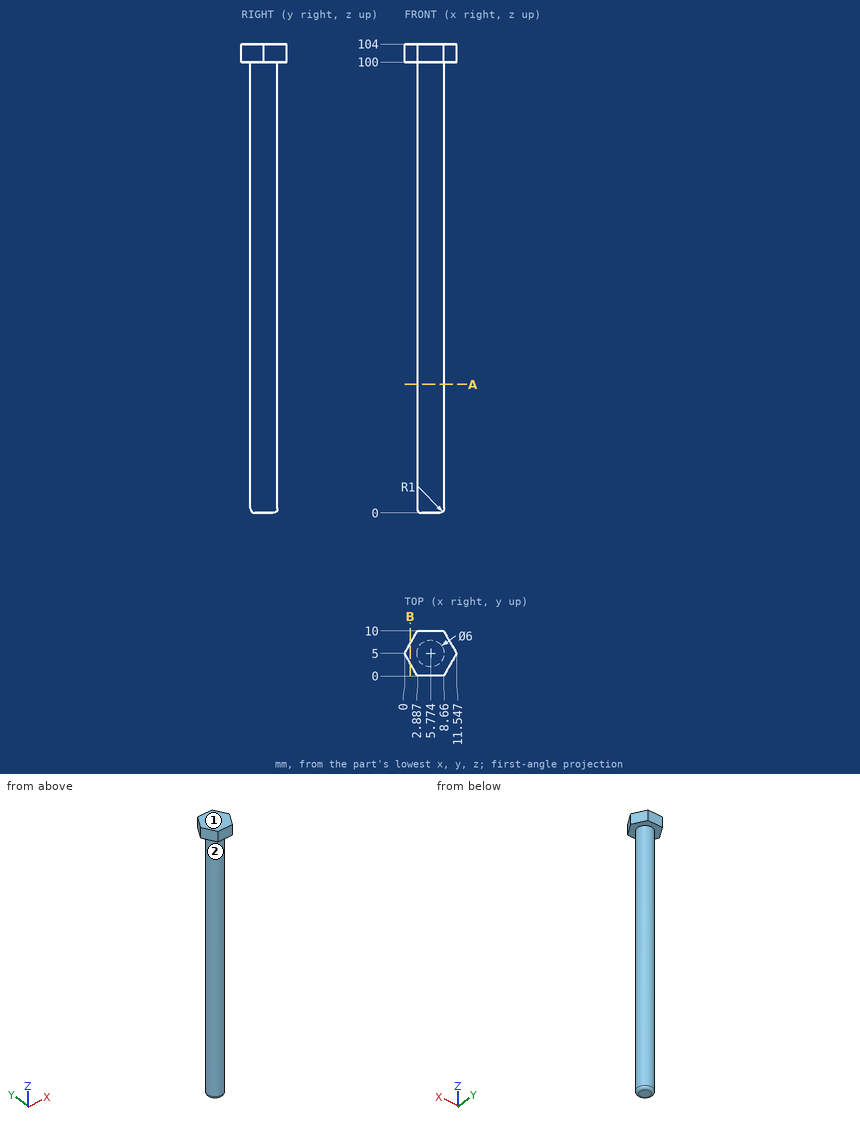
Design review of the part shown in the three views and the two pictorial views. Dimensions are in mm from the part's minimum x, y and z. A direction names the side the tool comes from. Give positions to 0.01 mm unless a question says otherwise; leave off trailing zeros. Write each loop counter-clockwise with the first axis right and the second up, starting at its lowest first coordinate (ties: lowest second). Pieces come first, ordered by that corner, then holes.
Item 1: Take a section at A-A (z = 28.5). Give the boundary of the cut face in (x, y), and give its area (3 significant figures).
Item 2: Take a section at B-B (x = 1.25). Give the boundary of the cut face in (y, z) (1 decimal).
Item 3: Machinability: for the marked faces 1 and 2, which of the approach directions +Z, -Z, +X, -X, +Y, -Y give a long, thin tool a straight path to every point of the face, cutting with its end or side? Answer none if there is none.
Item 4: Wall thickness on probe 1 along Z at (x, y) = (9, 7.5); probe 2 along X at (y, z) = (5.25, 33) (1 decimal); probe 3 along X at (y, z) = (2.75, 92) (1 decimal): over which ranges is each line inside the solid? List them lowest first.
Item 5: Insertion check: P1, Ø1.5, axis at y = 9, z = 26.5, coming from the -X side; P2, Ø3, axis at y = 5, z = 36.5, coming from the -X side; P3, Ø2, axis at y = 4.5, z = 36.5, coming from the +X side; P4, Ø1, axis at x = 8, z = 33, coming from the -Y side. Each pin has a flat end and moves straight along its axis. Give the tip position at first contact, or say it passes through.
Established:
1. outline: circle Ø6 at (5.77, 5)
1. area: 28.3 mm2
2. outline: (2.8, 100) - (7.2, 100) - (7.2, 104) - (2.8, 104) - close
3. face 1: +Z, +X, -X, +Y, -Y
3. face 2: -Z
4. probe 1: z = 100 to 104
4. probe 2: x = 2.8 to 8.8
4. probe 3: x = 3.8 to 7.8
5. P1: passes through
5. P2: stops at x = 2.77
5. P3: stops at x = 8.77
5. P4: stops at y = 2.55
